Autodesk Inventor part; units mm, degrees
ref_plane "YZ Plane" through (0, 0, 0) normal (1, 0, 0) x (0, 1, 0)
ref_plane "XZ Plane" through (0, 0, 0) normal (0, 1, 0) x (-1, 0, 0)
ref_plane "XY Plane" through (0, 0, 0) normal (0, 0, 1) x (1, 0, 0)
sketch "Sketch1" plane through (0, 0, 0) normal (0, 1, 0) x (-1, 0, 0)
  line L0 (20, 45) -> (-20, 45)
  line L1 (-20, 45) -> (-20, -45)
  line L2 (-20, -45) -> (20, -45)
  line L3 (20, -45) -> (20, 45)
  line L4 (20, 45) -> (-20, -45) construction
  line L5 (-20, 45) -> (20, -45) construction
  arc A0 (-20, -45) -> (20, -45) centre (0, -45) ccw
  line L6 (20, -45) -> (30, -45)
  line L7 (30, -45) -> (30, 45)
  line L8 (30, 45) -> (20, 45)
  line L9 (20, 45) -> (20, -45)
  point P0 (0, 0)
  dimension "d0" = 40
  dimension "d1" = 90
  dimension "d7" = 10
  dimension "d8" = 90
extrude "Extrusion1" add sketch "Sketch1" along normal blind 3.6
fillet "Fillet1" radius 4 3 edges at (-20, 1.8, -45) (-30, 1.8, -45) (20, 1.8, 45)
sketch "Sketch3" plane through (0, 0, 0) normal (0, -1, 0) x (1, 0, 0)
  circle A0 centre (0, -45) radius 21
  arc A1 (-19.7203, -48.3333) -> (20, -45) centre (0, -45) ccw
  point P0 (0, 0)
  dimension "d10" = 42
  dimension "d11" = 0
extrude "Extrusion3" cut sketch "Sketch3" against normal blind 10
fillet "Fillet2" radius 4 2 edges at (20, 1.8, -38.5969) (-20.9742, 1.8, -46.0397)
sketch "Sketch4" plane through (0, 0, 0) normal (0, -1, 0) x (1, 0, 0)
  circle A0 centre (-25.5, -40.5) radius 1.625
  line L0 (-24.6779, -45) -> (-26, -45)
  circle A1 centre (15.5, -19.5) radius 1.625
  circle A2 centre (15.5, 40.5) radius 1.625
  line L1 (20, 41) -> (20, -25.7906)
  arc A3 (13.44, -28.8641) -> (20, -25.7906) centre (16, -25.7906) ccw
  line L2 (-30, -41) -> (-30, 45)
  line L3 (-30, 45) -> (16, 45)
  point P0 (0, 0)
  point P1 (-30, 41)
  point P2 (-26, 45)
  dimension "d15" = 3.25
  dimension "d16" = 4.5
  dimension "d21" = 3.25
  dimension "d22" = 3.25
  dimension "d23" = 4.5
  dimension "d25" = 4.5
  dimension "d29" = 4.5
  dimension "d30" = 4.5
  dimension "d31" = 60
extrude "Extrusion4" cut sketch "Sketch4" against normal blind 7
sketch "Sketch5" plane through (0, 0, 0) normal (0, -1, 0) x (1, 0, 0)
  line L0 (-15.5, 30) -> (5.5, 30)
  line L1 (5.5, 30) -> (5.5, -13)
  line L2 (5.5, -13) -> (-15.5, -13)
  line L3 (-15.5, -13) -> (-15.5, 30)
  line L4 (-15.5, 30) -> (5.5, -13) construction
  line L5 (5.5, 30) -> (-15.5, -13) construction
  line L6 (-24.6779, -45) -> (-26, -45)
  line L7 (-30, -41) -> (-30, 45)
  point P0 (0, 0)
  point P1 (-5, 8.5)
  point P2 (-30, 41)
  dimension "d32" = 21
  dimension "d33" = 43
  dimension "d34" = 32
  dimension "d35" = 14.5
extrude "Extrusion5" cut sketch "Sketch5" against normal blind 10
sketch "Sketch6" plane through (0, 0, 0) normal (0, -1, 0) x (1, 0, 0)
  circle A0 centre (0, -18) radius 2.5
  circle A1 centre (0, 33) radius 2.5
  circle A2 centre (-10, -18) radius 2.5
  circle A3 centre (-10, 33) radius 2.5
  line L0 (5.5, 30) -> (5.5, -13)
  line L1 (5.5, -13) -> (-15.5, -13)
  point P0 (0, 0)
  dimension "d38" = 5
  dimension "d39" = 5
  dimension "d40" = 51
  dimension "d41" = 5
  dimension "d42" = 5
  dimension "d43" = 10
  dimension "d44" = 10
  dimension "d45" = 51
  dimension "d46" = 90
  dimension "d47" = 5.5
  dimension "d48" = 5
extrude "Extrusion6" cut sketch "Sketch6" against normal blind 10
fillet "Fillet3" radius 25 1 edges at (-30, 1.8, 45)
properties part number "p1"
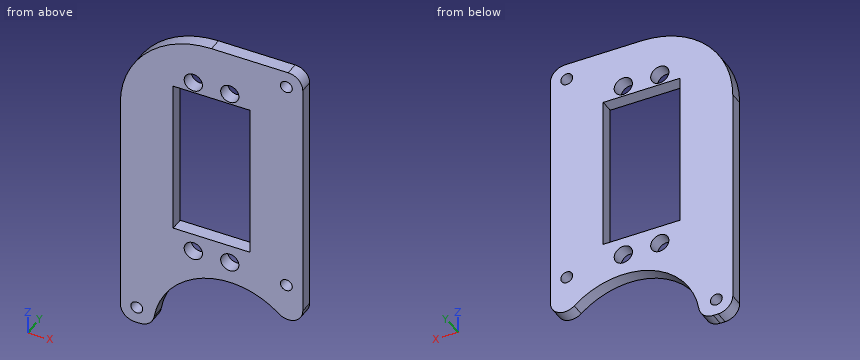
Check sheet for the modelled part. Datum: model origin and axes. Units: mm. Round coordinates to 2 decimals unless told otherwise and drop trailing zeros. Order: outer loops, then holes, each group sorted by start corner. A loop starts at its lowest first (then second) coordinate and runs counter-clockwise, first axis right, second up.
(1) Scan lines: probe 1 along Z at (x, y) = (0, 1.2); probe 2 along X at (y, z) = (1.1, -10); probe 3 along Z at (x, y) = (2, 2.5). Record each from-to range of solid material in increasing order.
(2) Cross-section at B-B, the plane z = 11.5. Enter the section's corners in (x, y).
(3) Cross-section at C-C, the plane z = 33. Enter the section's corners in (x, y), and give its area (3 significant figures).
(4) Cross-section at D-D, the plane y = 2.85. State how many separate pieces and enclosed holes the cut face has, and give its area (3 significant figures).
(5) Go/stop test with flat-tipped pins: P1, Ø3.5, axis at x = 15.5, z = -19.5, coming from the -Y side; P2, Ø1.5, axis at x = -8.5, y = 1, coming from the -Z side; P3, Ø2, axis at x = -12.5, y = 2.5, coming from the +Z side; P4, Ø1.1, axis at x = -5.5, y = 1.5, coming from the -Z side. Record where each tip stops, or that it passes through.
(6) Cross-section at A-A, the plane x = 0. Enter the section's corners in (y, z), and give its area (3 significant figures).
Check sheet entries:
1. probe 1: z = -24 to -20.5, -15.5 to -13, 30 to 30.5, 35.5 to 45
1. probe 2: x = -30 to -15.5, 5.5 to 20
1. probe 3: z = -24.1 to -19.5, -16.5 to -13, 30 to 31.5, 34.5 to 45
2. outline: (-30, 0) - (-15.5, 0) - (-15.5, 3.6) - (-30, 3.6) - close; (5.5, 0) - (20, 0) - (20, 3.6) - (5.5, 3.6) - close
3. outline: (-26.35, 0) - (-12.5, 0) - (-12.5, 3.6) - (-26.35, 3.6) - close; (-7.5, 0) - (-2.5, 0) - (-2.5, 3.6) - (-7.5, 3.6) - close; (2.5, 0) - (20, 0) - (20, 3.6) - (2.5, 3.6) - close
3. area: 131 mm2
4. separate pieces: 1
4. enclosed holes: 8
4. area: 2,640 mm2
5. P1: stops at y = 0
5. P2: stops at z = -26.15
5. P3: stops at z = 44.14
5. P4: stops at z = -24.89
6. outline: (0, -24) - (3.6, -24) - (3.6, -20.5) - (0, -20.5) - close; (0, -15.5) - (3.6, -15.5) - (3.6, -13) - (0, -13) - close; (0, 30) - (3.6, 30) - (3.6, 30.5) - (0, 30.5) - close; (0, 35.5) - (3.6, 35.5) - (3.6, 45) - (0, 45) - close
6. area: 57.6 mm2
